Job drawing, mm, ordinate dimensions from the low corner. One solid piece. A direction names the side the tool comes from. Round coordinates to 2 decimals unless told otherwise and drop trailing zeros. Order: outer loops, then holes, each group sorted by start corner. A loop starts at its lowest first (then second) coordinate and runs counter-clockwise, first axis right, second up. Notation, with made-up numbers: (52.5, 19) -> (57.5, 19) arc R13 cw to (57.5, 24) -> close; hole circle Ø3 at (22, 25.25). An arc over 180 degrees is marked (long way). Write item = value, one per line.
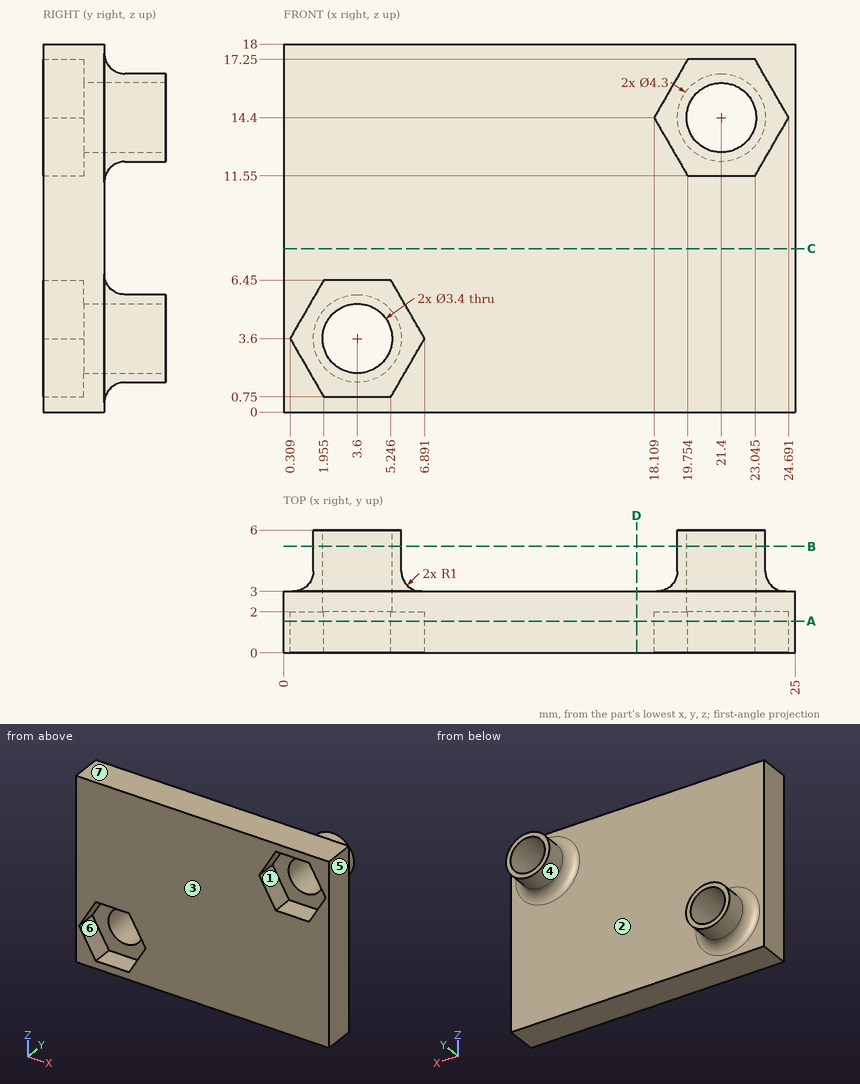
Q1. Cut at C-C, the plane z = 8. List the corners of the cut face in (x, y).
Check values:
outline = (0, 0) -> (25, 0) -> (25, 3) -> (0, 3) -> close
Q2. Mould opens along X. For the marked faces 4, 5, 6 and 7 say: released by +X, released by -X, zero draft, split by the parting line, or undercut.
Check values:
face_4 = split by the parting line
face_5 = released by +X
face_6 = undercut
face_7 = zero draft
Q3. Cut at B-B, the plane y = 5.2. List the corners of the cut face in (x, z).
Check values:
outline = circle Ø4.3 at (3.6, 3.6); circle Ø4.3 at (21.4, 14.4); hole circle Ø3.4 at (3.6, 3.6); hole circle Ø3.4 at (21.4, 14.4)
Q4. Cut at A-A, the plane y = 1.55. Give the number of separate pieces and of enclosed holes in the cut face, and give its area (3 significant figures).
Check values:
separate_pieces = 1
enclosed_holes = 2
area = 394 mm²
Q5. Cut at D-D, the plane x = 17.25. List the corners of the cut face in (y, z), and give its area (3 significant figures).
Check values:
outline = (0, 0) -> (3, 0) -> (3, 18) -> (0, 18) -> close
area = 54.0 mm²
Q6. Flat gauge pins, fed straight in: pin 1 (2 mm diameter, centred on x = 3.6, z = 3.6, fed in from +Y); pin 2 (2 mm diameter, centred on x = 19.5, y = 4.5, fed in from -Z); pin 3 (3 mm diameter, centred on x = 22, z = 15.5, fed in from -Y). Where does each tip first touch, or does it go through?
Check values:
pin_1 = through
pin_2 = 12.45
pin_3 = 2
Q7. Probe probe 1 along Z at (x, y) = (21.75, 1.35); probe 2 along Y at (x, z) = (1.75, 15.5); probe 3 along Z at (x, y) = (21, 5.4). List the from-to ranges inside material, lowest first.
Check values:
probe_1 = 0 to 11.55, 17.25 to 18
probe_2 = 0 to 3
probe_3 = 12.29 to 12.75, 16.05 to 16.51
Q8. Which spindle directions (+Z, -Z, +X, -X, +Y, -Y) get a long thin tool onto all of the face, cutting with end or side? Do the marked faces 1, 2 and 3. Say none if no direction does.
Check values:
face_1 = -Y
face_2 = +Y
face_3 = +Z, -Z, +X, -X, -Y
